from build123d import *

# Parameters (mm, degrees)
EXTRUSION1_DEPTH             = 14
EXTRUSION1_DEPTH_BACK        = 2
ESQUISSE2_R                  = 19.8
ESQUISSE2_R_2                = 15
CONG_1_R                     = 1
CHANFREIN1_SIZE              = 0.5
ESQUISSE5_W                  = 2.5
ESQUISSE5_H                  = 19.8
R_P_TITION_CIRCULAIRE1_COUNT = 2
R_P_TITION_CIRCULAIRE1_ANGLE = 90


with BuildPart() as part:
    # Esquisse1 → Base-R_volution (revolve)
    with BuildSketch(Plane(origin=(0, 0, 0), x_dir=(1, 0, 0), z_dir=(0, 1, 0)), mode=Mode.PRIVATE) as base_r_volution_sk:
        with BuildLine():
            Line((0, 19.8), (0, 16))
            ThreePointArc((0, 16), (0.292893219, 15.292893219), (1, 15))
            Line((1, 15), (15, 15))
            ThreePointArc((15, 15), (15.707106781, 15.292893219), (16, 16))
            Line((16, 16), (16, 19.8))
            Line((16, 19.8), (11.577708764, 19.8))
            ThreePointArc((11.577708764, 19.8), (8, 18.2), (4.422291236, 19.8))
            Line((4.422291236, 19.8), (0, 19.8))
        make_face()
    revolve(base_r_volution_sk.sketch.rotate(Axis((0, 0, 0), (1, 0, 0)), 180), axis=Axis((0, 0, 0), (1, 0, 0)))

    # Esquisse2 → Extrusion1 (add, two sides: drawn at the far end of the back side and taken through both)
    with BuildSketch(Plane.ZY.offset(-EXTRUSION1_DEPTH_BACK)):
        Circle(ESQUISSE2_R)
        Circle(ESQUISSE2_R_2, mode=Mode.SUBTRACT)
    extrude(amount=EXTRUSION1_DEPTH + EXTRUSION1_DEPTH_BACK)

    # Cong_1
    cong_1_edges = [part.edges().sort_by_distance(p)[0] for p in [
        (-14, 0, -15),
    ]]
    fillet(cong_1_edges, radius=CONG_1_R)

    # Chanfrein1
    chanfrein1_edges = [part.edges().sort_by_distance(p)[0] for p in [
        (-14, 0, -19.8),
    ]]
    chamfer(chanfrein1_edges, length=CHANFREIN1_SIZE)

    # Esquisse5 → Trou taraud_ M61 (revolve, cut)
    with BuildSketch(Plane(origin=(-8, 0, 0), x_dir=(0, 0, -1), z_dir=(1, 0, 0))):
        with Locations((1.25, 9.9)):
            Rectangle(ESQUISSE5_W, ESQUISSE5_H)
    trou_taraud_m61 = revolve(axis=Axis((-8, -6.35, 0), (0, 1, 0)), mode=Mode.SUBTRACT)

    # R_p_tition circulaire1: Trou taraud_ M61 ×2 about axis
    r_p_tition_circulaire1_axis = Axis((15, 0, 0), (-1, 0, 0))
    for i in range(1, R_P_TITION_CIRCULAIRE1_COUNT):
        add(trou_taraud_m61.rotate(r_p_tition_circulaire1_axis, i * R_P_TITION_CIRCULAIRE1_ANGLE / (R_P_TITION_CIRCULAIRE1_COUNT - 1)), mode=Mode.SUBTRACT)


solid = part.part
Geometry check sheet. Reference: the model listing, model coordinates, mm. A direction names the side the tool comes from. Round coordinates to 2 decimals unless told otherwise and drop trailing zeros. Order: outer loops, then holes, each group sorted by start corner. A loop starts at its lowest first (then second) coordinate and runs counter-clockwise, first axis right, second up. Notation, with made-up numbers: M 83.25,-34 L 115.25,-34 A37 cw 115.25,3 Z; hole C 9.5,61 d11. An arc over 180 degrees is marked long. Answer in a Markdown table with one row per item. Add a question column.
Item 1: Draft check along X on faces 1 (the face through (-5.56, 17.33, 0.54)), 2 (the face through (16, 15, -7)), 3 (the face through (13.8, -5.9, 18.9)). Enter one of: released by +X, released by -X, zero draft, split by the parting line, or undercut.
Item 2: Sectioned sample at D-D, the plane x = 13.5. Enter the section's corners in (y, z).
Item 3: Set-up check for faces 4 (the face through (-5.56, 0.54, -17.33)), 5 (the face through (-14, 16, 3)): record each of +Z, -Z, +X, -X, +Y, -Y from which the full face is reachable in a straight line by a thin tool's end or side.
Item 4: Sectioned sample at A-A, the plane y = 0. Enter the section's corners in (x, z).
Item 5: Depth check by flat-ended pin: pin 1 Ø1 at (x, z) = (4.5, -6.5) entering from +Y; pin 2 Ø3 at (x, z) = (-8, 0) entering from +Y; pin 3 Ø8 at (y, z) = (9, -10.5) entering from +X; pin 4 Ø4 at (x, y) = (-8, 0) entering from -Z. Enter the tip coordinate at first touch or a pass-through.
Item 6: Material ranges on L1, parallel to Z at x = -7.75, y = 0; L2, parallel to Y at x = 7, z = -1; L3, parallel to Y at x = 12, z = 0, recorded low to high. Write a range as [from, to].
Item 7: Sectioned sample at B-B, the plane z = 0. Enter the section's corners in (x, y).
Item 8: Sectioned sample at C-C, the plane x = -8. Enter the section's corners in (y, z), plus the area to 3 significant figures.
Filled in:
| question | item | result |
|---|---|---|
| 1 | face 1 | undercut |
| 1 | face 2 | released by +X |
| 1 | face 3 | zero draft |
| 2 | outline | C 0,0 d39.6; hole C 0,0 d30 |
| 3 | face 4 | -Z |
| 3 | face 5 | +Z, -Z, -X, +Y, -Y |
| 4 | outline | M -14,-19.3 L -13.5,-19.8 L -10.5,-19.8 L -10.5,-15 L -13,-15 A1 ccw -14,-16 Z; M -14,16 A1 ccw -13,15 L 15,15 A1 ccw 16,16 L 16,19.8 L 11.58,19.8 A4.8 cw 4.42,19.8 L -13.5,19.8 L -14,19.3 Z; M -5.5,-19.8 L 4.42,-19.8 A4.8 cw 11.58,-19.8 L 16,-19.8 L 16,-16 A1 ccw 15,-15 L -5.5,-15 Z |
| 5 | pin 1 | stops at y = 18.87 |
| 5 | pin 2 | stops at y = -14.92 |
| 5 | pin 3 | stops at x = 16 |
| 5 | pin 4 | stops at z = 14.87 |
| 6 | L1 | z = [15, 19.8] |
| 6 | L2 | y = [-18.28, -14.97], [14.97, 18.28] |
| 6 | L3 | y = [-19.8, -15], [15, 19.8] |
| 7 | outline | M -14,-19.3 L -13.5,-19.8 L 4.42,-19.8 A4.8 cw 11.58,-19.8 L 16,-19.8 L 16,-16 A1 ccw 15,-15 L -13,-15 A1 ccw -14,-16 Z; M -14,16 A1 ccw -13,15 L -10.5,15 L -10.5,19.8 L -13.5,19.8 L -14,19.3 Z; M -5.5,15 L 15,15 A1 ccw 16,16 L 16,19.8 L 11.58,19.8 A4.8 cw 4.42,19.8 L -5.5,19.8 Z |
| 8 | outline | M -2.5,-19.64 L -2.5,-14.79 A15 cw long 14.79,2.5 L 19.64,2.5 A19.8 ccw long Z; M 2.5,-19.64 A19.8 ccw 19.64,-2.5 L 14.79,-2.5 A15 cw 2.5,-14.79 Z |
| 8 | area | 477 mm² |
